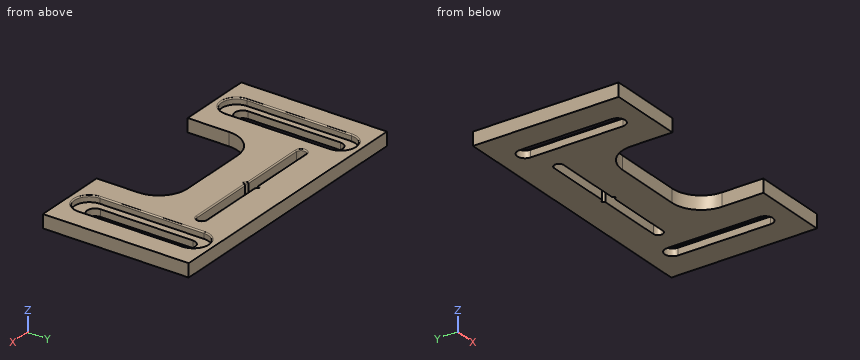
```python
from build123d import *

# Parameters (mm, degrees)
PAD_DEPTH    = 11.25
POCKET_DEPTH = 5.25
FILLET_R     = 1


with BuildPart() as part:
    # Sketch → Pad (new body)
    with BuildSketch(Plane.XY):
        with BuildLine():
            Line((117.4, 123.025), (117.4, 0))
            Line((117.4, 0), (53.9, 0))
            Line((53.9, 0), (53.9, 35))
            ThreePointArc((53.9, 35), (46.716794, 52.341794), (29.375, 59.525))
            Line((29.375, 59.525), (-29.375, 59.525))
            ThreePointArc((-29.375, 59.525), (-46.716794, 52.341794), (-53.9, 35))
            Line((-53.9, 35), (-53.9, 0))
            Line((-53.9, 0), (-117.4, 0))
            Line((-117.4, 0), (-117.4, 123.025))
            Line((-117.4, 123.025), (117.4, 123.025))
        make_face()
        with BuildLine():
            ThreePointArc((-80.8875, 100.525), (-87.3875, 107.025), (-93.8875, 100.525))
            Line((-93.8875, 100.525), (-93.8875, 22.5))
            ThreePointArc((-93.8875, 22.5), (-87.3875, 16), (-80.8875, 22.5))
            Line((-80.8875, 22.5), (-80.8875, 100.525))
        make_face(mode=Mode.SUBTRACT)
        with BuildLine():
            ThreePointArc((93.8875, 100.525), (87.3875, 107.025), (80.8875, 100.525))
            Line((80.8875, 100.525), (80.8875, 22.5))
            ThreePointArc((80.8875, 22.5), (87.3875, 16), (93.8875, 22.5))
            Line((93.8875, 22.5), (93.8875, 100.525))
        make_face(mode=Mode.SUBTRACT)
        with BuildLine():
            ThreePointArc((-58.7, 96.26875), (-62.7, 92.26875), (-58.7, 88.26875))
            Line((-58.7, 88.26875), (-2, 88.26875))
            Line((-2, 88.26875), (0, 86.26875))
            Line((0, 86.26875), (2, 88.26875))
            Line((2, 88.26875), (58.7, 88.26875))
            ThreePointArc((58.7, 88.26875), (62.7, 92.26875), (58.7, 96.26875))
            Line((58.7, 96.26875), (2, 96.26875))
            Line((0, 98.26875), (2, 96.26875))
            Line((-2, 96.26875), (0, 98.26875))
            Line((-2, 96.26875), (-58.7, 96.26875))
        make_face(mode=Mode.SUBTRACT)
    extrude(amount=PAD_DEPTH)

    # Sketch001 (on Face30 of Pad) → Pocket (cut)
    with BuildSketch(Plane.XY.offset(11.25)):
        with BuildLine():
            ThreePointArc((-74.6375, 105.525), (-87.1375, 118.025), (-99.6375, 105.525))
            Line((-99.6375, 105.525), (-99.6375, 17.5))
            ThreePointArc((-99.6375, 17.5), (-87.1375, 5), (-74.6375, 17.5))
            Line((-74.6375, 17.5), (-74.6375, 105.525))
        make_face()
        with BuildLine():
            ThreePointArc((99.6375, 105.525), (87.1375, 118.025), (74.6375, 105.525))
            Line((74.6375, 105.525), (74.6375, 17.5))
            ThreePointArc((74.6375, 17.5), (87.1375, 5), (99.6375, 17.5))
            Line((99.6375, 17.5), (99.6375, 105.525))
        make_face()
    extrude(amount=-POCKET_DEPTH, mode=Mode.SUBTRACT)

    # Fillet
    fillet_edges = [part.edges().sort_by_distance(p)[0] for p in [
        (30.35, 96.26875, 11.25),
        (62.7, 92.26875, 11.25),
        (30.35, 88.26875, 11.25),
        (1, 87.26875, 11.25),
        (-1, 87.26875, 11.25),
        (1, 97.26875, 11.25),
        (-1, 97.26875, 11.25),
        (-30.35, 96.26875, 11.25),
        (-30.35, 88.26875, 11.25),
        (-62.7, 92.26875, 11.25),
        (-74.6375, 61.5125, 11.25),
        (-87.1375, 118.025, 11.25),
        (-99.6375, 61.5125, 11.25),
        (87.1375, 118.025, 11.25),
        (74.6375, 61.5125, 11.25),
        (99.6375, 61.5125, 11.25),
        (87.1375, 5, 11.25),
        (-87.1375, 5, 11.25),
    ]]
    fillet(fillet_edges, radius=FILLET_R)


solid = part.part
```
Part model, mm, in its own coordinate system. Give positions to 0.01 mm unless a question says otherwise; leave off trailing zeros. Order: outer loops, then holes, each group sorted by start corner. A loop starts at its lowest first (then second) coordinate and runs counter-clockwise, first axis right, second up. Notation, with made-up numbers: (75, -10.5) - (118, -10.5) arc R27 ccw to (118, 8.5) - close; hole circle Ø7 at (87.25, 82). An arc over 180 degrees is marked (long way). Use one line per item in the form item = value.
Item 1: Probe probe 1 along X at (y, z) = (102.5, 6.25); probe 2 along X at (y, z) = (22.5, 2.5); probe 3 along Y at (x, z) = (-14, 10) (3 decimals). List the from-to ranges inside material, lowest first. Write a range as from..to.
Solution:
probe_1 = -117.4..-99.64, -74.64..74.64, 99.64..117.4
probe_2 = -117.4..-93.89, -80.89..-53.9, 53.9..80.89, 93.89..117.4
probe_3 = 59.525..88.269, 96.269..123.025
Item 2: Slice it at B-B on x = 5. Give the cut face in (y, z) (3 decimals), and give its area (3 significant figures).
Solution:
outline = (59.525, 0) - (88.269, 0) - (88.269, 10.25) arc R1 ccw to (87.269, 11.25) - (59.525, 11.25) - close; (96.269, 0) - (123.025, 0) - (123.025, 11.25) - (97.269, 11.25) arc R1 ccw to (96.269, 10.25) - close
area = 624 mm2
Item 3: Slice it at A-A on z = 8. Count the separate pieces of the cut face and the enclosed holes in it, and give its area (3 significant figures).
Solution:
separate_pieces = 1
enclosed_holes = 3
area = 16,300 mm2
Item 4: Pin check, flat tips, straight feed: pin 1 Ø7.5 at (x, y) = (-89.5, 49.5) entering from +Z (3 decimals); pin 2 Ø3 at (x, z) = (23.5, 6.5) entering from -Y (3 decimals); pin 3 Ø5 at (x, z) = (-29.5, 6.5) entering from -Y. Stop position of each tip, or through.
Solution:
pin_1 = through
pin_2 = 59.525
pin_3 = 59.38
